from build123d import *

# Parameters (mm, degrees)
SKETCH1_R           = 10
BOSS_EXTRUDE1_DEPTH = 60
CUT_EXTRUDE1_START  = -17.384625528
CUT_EXTRUDE1_DEPTH  = 30
SKETCH3_R           = 10
BOSS_EXTRUDE2_DEPTH = 26.2874406
BOSS_EXTRUDE3_START = 26.2874406
SKETCH4_R           = 10
BOSS_EXTRUDE3_DEPTH = 26.2874406


# Read off the part's stored shape, not the designer's step: Cut-Extrude1
with BuildPart() as part:
    # Sketch1 → Boss-Extrude1 (new body)
    # profile 1 of 3: a face of its own
    with BuildSketch(Plane.XY):
        with BuildLine():
            Line((-81.993392368, 14.695588132), (-85, 15))
            ThreePointArc((-85, 15), (-100, 0), (-85, -15))
            Line((-85, -15), (-81.993392368, -14.695588132))
            ThreePointArc((-81.993392368, -14.695588132), (-73.378917553, -9.484220725), (-70, 0))
            ThreePointArc((-70, 0), (-73.378917553, 9.484220725), (-81.993392368, 14.695588132))
        make_face()
        with Locations(Location((-85, 0, 0), (0, 0, 180))):
            Circle(SKETCH1_R, mode=Mode.SUBTRACT)
    # profile 2 of 3: a face of its own
    with BuildSketch(Plane.XY):
        with BuildLine():
            Line((39.599219547, 2.384625528), (-81.993392368, 14.695588132))
            ThreePointArc((-81.993392368, 14.695588132), (-73.378917553, 9.484220725), (-70, 0))
            ThreePointArc((-70, 0), (-73.378917553, -9.484220725), (-81.993392368, -14.695588132))
            Line((-81.993392368, -14.695588132), (39.599219547, -2.384625528))
            Line((39.599219547, -2.384625528), (80.215221564, -2.384625528))
            ThreePointArc((80.215221564, -2.384625528), (80.005468162, 0.009549459), (80.373005951, 2.384625528))
            Line((80.373005951, 2.384625528), (66.359528771, 2.384625528))
            Line((66.359528771, 2.384625528), (39.599219547, 2.384625528))
        make_face()
    # profile 3 of 3: a face of its own
    with BuildSketch(Plane.XY):
        with Locations((90, -0.321106458)):
            Circle(SKETCH1_R)
    extrude(amount=BOSS_EXTRUDE1_DEPTH)

    # Cut-Extrude1 outline → Cut-Extrude1 (cut)
    with BuildSketch(Plane(origin=(0, 2.384625528, 0), x_dir=(1, 0, 0), z_dir=(0, 1, 0)).offset(CUT_EXTRUDE1_START)):
        Polygon((34.734743134, -25), (80.373005951, -25), (80.373005951, -3.7125594), (101, -3.7125594), (101, 0), (26.666623154, 0), align=None)
        Polygon((101, -60), (101, -56.2874406), (80.373005951, -56.2874406), (80.373005951, -35), (34.734743134, -35), (26.666623154, -60), align=None)
        Polygon((-5.086975799, -7.68377667), (-101, -7.68377667), (-101, -52.31622333), (-5.086975799, -52.31622333), (17.229247531, -30), align=None)
    extrude(amount=CUT_EXTRUDE1_DEPTH, mode=Mode.SUBTRACT)

    # Sketch3 → Boss-Extrude2 (add)
    with BuildSketch(Plane.XY.offset(56.2874406)):
        with Locations(Location((90, -0.321106458, 0), (0, 0, 191.908649851))):
            Circle(SKETCH3_R)
    extrude(amount=BOSS_EXTRUDE2_DEPTH)

    # Sketch4 → Boss-Extrude3 (add)
    with BuildSketch(Plane(origin=(0, 0, 3.7125594), x_dir=(-1, 0, 0), z_dir=(0, 0, -1)).offset(BOSS_EXTRUDE3_START)):
        with Locations((-90, -0.321106458)):
            Circle(SKETCH4_R)
    extrude(amount=-BOSS_EXTRUDE3_DEPTH)


solid = part.part
The listing builds one solid part. Answer for the finished solid, in the listing's coordinates (mm). A direction names the side the tool comes from. Round coordinates to 2 decimals unless told otherwise and drop trailing zeros. Write each loop counter-clockwise with the first axis right and the second up, starting at its lowest first coordinate (ties: lowest second). Pieces come first, ordered by that corner, then holes. Notation, with made-up numbers: (-8, 28.5) - (6, 28.5) arc R12 ccw to (6, 51.5) - close; hole circle Ø3 at (6.25, 70.5). An arc over 180 degrees is marked (long way). Use a Markdown table: item, result. Add a question column.
1. A tool of negligible diameter and unlimited length cuts with its end or side. For faces 5 (the face through (80.373, 0, 46)), 6 (the face through (60, 2.385, 30)), 7 (the face through (30.76, -0.05, 47.32)), 8 (the face through (-53, 0, 52.316)), from which of +Z, -Z, +X, -X, +Y, -Y can it reach the whole face along a straight path? Write none if from no direction.
2. For a pull along Z with two mould halves and no side action, classify faces 1 (the face through (6.23, -0.1, 19)), 2 (the face through (-100, 0, 4)), 3 (the face through (5.915, -0.097, 41.314)), 4 (the face through (90, 0, -22.575)) as +Z half, -Z half, draft (parallel to the pull), parting line (faces both ways), or undercut.
3. The part is cut by section D-D (z = 76.5). Write down the section's boundary in (x, y).
4. Consider line 1 (Z direction, x = -63.5, y = -9.5); line 2 (Y direction, x = -85, z = 3.25); line 3 (Z direction, x = 24, y = -2.25). Determine where each line is inside the solid, lowest interval first.
5. The part is cut by section A-A (y = 12.5). Write down the section's boundary in (x, z).
6. The part is cut by section C-C (x = 90). Write down the section's boundary in (y, z), and give its area (3 significant figures).
7. The part is cut by section B-B (z = 49). Write down the section's boundary in (x, y).
8. Flat-ended cylindrical pins translate along their axes: P1, Ø3, axis at x = 58, y = 1, coming from the -Z side; P2, Ø1.8, axis at x = 60, y = -1, coming from the +Z side; P3, Ø1, axis at x = -21, z = 1, coming from the +Y side. Find the tip coordinate at first contact, or state that the pin passes through.
Reported:
| question | item | result |
|---|---|---|
| 1 | face 5 | +Y, -Y |
| 1 | face 6 | +Z, -Z, +Y |
| 1 | face 7 | +Z, +Y, -Y |
| 1 | face 8 | -X, +Y, -Y |
| 2 | face 1 | undercut |
| 2 | face 2 | draft |
| 2 | face 3 | undercut |
| 2 | face 4 | -Z half |
| 3 | outline | circle Ø20 at (90, -0.32) |
| 4 | line 1 | 0 to 7.68, 52.32 to 60 |
| 4 | line 2 | -15 to -10, 10 to 15 |
| 4 | line 3 | 0 to 60 |
| 5 | outline | (-93.29, 0) - (-60.31, 0) - (-60.31, 7.68) - (-93.29, 7.68) - close; (-93.29, 52.32) - (-60.31, 52.32) - (-60.31, 60) - (-93.29, 60) - close |
| 6 | outline | (-10.32, -22.57) - (9.68, -22.57) - (9.68, 82.57) - (-10.32, 82.57) - close |
| 6 | area | 2,100 mm^2 |
| 7 | outline | (-1.77, -6.57) - (30.22, -3.33) - (30.22, 3.33) - (-1.77, 6.57) - close; (80.37, -3.03) arc R10 ccw (long way) to (80.37, 2.38) - close |
| 8 | P1 | z = 25 |
| 8 | P2 | z = 35 |
| 8 | P3 | y = 8.57 |
